Autodesk Inventor part; units mm, degrees
ref_plane "YZ Plane" through (0, 0, 0) normal (1, 0, 0) x (0, 1, 0)
ref_plane "XZ Plane" through (0, 0, 0) normal (0, 1, 0) x (-1, 0, 0)
ref_plane "XY Plane" through (0, 0, 0) normal (0, 0, 1) x (1, 0, 0)
sketch "スケッチ1" plane through (0, 0, 0) normal (0, 1, 0) x (-1, 0, 0)
  circle A0 centre (0, 0) radius 6
  dimension "d0" = 12
extrude "押し出し1" add sketch "スケッチ1" along normal blind 8.5
sketch "スケッチ2" plane through (0, 0, 0) normal (0, -1, 0) x (1, 0, 0)
  circle A0 centre (0, 0) radius 3.25
  line L0 (-5.9563, 0) -> (5.7903, 0)
  circle A1 centre (-3.25, 0) radius 0.25
  circle A2 centre (3.25, 0) radius 0.25
  dimension "d3" = 6.5
  dimension "d4" = 0.5
  dimension "d5" = 0.5
extrude "押し出し2" add sketch "スケッチ2" along normal blind 5 contours L0 A2 A0 | L0 A2 A0 | A0 A2 L0 | A0 A2 L0 | A1 L0 A0 | A0 L0 A1 | A1 L0 A0 | A0 L0 A1
properties part number "Buzzer"
Part model, mm, in its own coordinate system. Round coordinates to 2 decimals unless told otherwise and drop trailing zeros. Write each loop counter-clockwise with the first axis right and the second up, starting at its lowest first coordinate (ties: lowest second). Pieces come first, ordered by that corner, then holes. Notation, with made-up numbers: M -32.75,78.25 L 16.25,78.25 A17 ccw 16.25,107.25 Z; hole C 62.5,-12 d5. An arc over 180 degrees is marked long. Answer as CSV lines item,"result". Start each with the question number.
1) Band-saw the part on D-D (y = 2.25). List the corners of the cut face in (x, z).
2) Drill centre lines: L1, parallel to Y at x = 0.25, z = -1; L2, parallel to X at y = 5.25, z = -1; L3, parallel to X at y = 1, z = -4. Where is each one in solid material? Low to high.
3) Band-saw the part on C-C (x = 0). List the corners of the cut face in (y, z).
4) Band-saw the part on A-A (y = -0.25). List the corners of the cut face in (x, z), then the cut area to 3 significant figures.
5) Drop flat-ended pins along their axis: pin 1 (6 mm diameter, centred on x = -2, z = 0.5, fed in from -Y); pin 2 (3 mm diameter, centred on x = -3, z = 3, fed in from -Y); pin 3 (1 mm diameter, centred on y = 6, z = 3, fed in from -X). Give the stop position or say it passes through.
6) Band-saw the part on B-B (z = 0). List the corners of the cut face in (x, y).
Worked out:
1,outline,"C 0,0 d12"
2,L1,"0 to 8.5"
2,L2,"-5.92 to 5.92"
2,L3,"-4.47 to 4.47"
3,outline,"M 0,-6 L 8.5,-6 L 8.5,6 L 0,6 Z"
4,outline,"C -3.25,0 d0.5; C 3.25,0 d0.5"
4,area,"0.393 mm²"
5,pin 1,"y = -5"
5,pin 2,"y = 0"
5,pin 3,"x = -5.45"
6,outline,"M -6,0 L -3.5,0 L -3.5,-5 L -3,-5 L -3,0 L 3,0 L 3,-5 L 3.5,-5 L 3.5,0 L 6,0 L 6,8.5 L -6,8.5 Z"
